The drawing under review shows one solid part. Ordinate dimensions are in mm from its lowest x, y, z. A direction names the side the tool comes from. Give positions to 0.01 mm unless a question says otherwise; leave off trailing zeros. Order: outer loops, then holes, each group sorted by start corner. A loop starts at its lowest first (then second) coordinate and runs counter-clockwise, first axis right, second up. Notation, with made-up numbers: (50.5, -21) - (94.5, -21) arc R25 cw to (94.5, 17) - close; hole circle Ø8 at (33.25, 8). An arc over 180 degrees is marked (long way). Write item = value, one per line. Start each with the question number.
1. Wall thickness on probe 1 along X at (y, z) = (3.75, 15.65); probe 2 along Z at (x, y) = (25, 6); probe 3 along Z at (x, y) = (11.5, 4.75): over which ranges is each line inside the solid? List them lowest first.
2. We need section C-C, the plane y = 4.25. State how many separate pieces and enclosed holes the cut face has.
3. Mouldability with a two-part tool opening along Z and no side actions: class the marked faces 5, 6 and 7 as pulls with the +Z half, pulls with the -Z half, needs draft (parallel to the pull), parting line crosses it, or undercut.
4. Machinability: for the marked faces 1, 2, 3 and 4, which of the approach directions +Z, -Z, +X, -X, +Y, -Y give a long, thin tool a straight path to every point of the face, cutting with its end or side? Answer none if there is none.
5. We need section D-D, the plane z = 8.5. Give the boundary of the cut face in (x, y).
6. We need section B-B, the plane z = 5.35. Give the boundary of the cut face in (x, y), and give its area (3 significant figures).
7. We need section A-A, the plane x = 25.1. Give the boundary of the cut face in (y, z).
8. For P1, Ø1.5, axis at x = 31, y = 1, coming from the -Z side; P2, Ø6, axis at y = 3.5, z = 4.5, coming from the +X side; P3, Ø1.6, axis at y = 5.5, z = 1.5, coming from the -X side, all flat-tipped, find the tip position at first contact; note any pin that passes through.
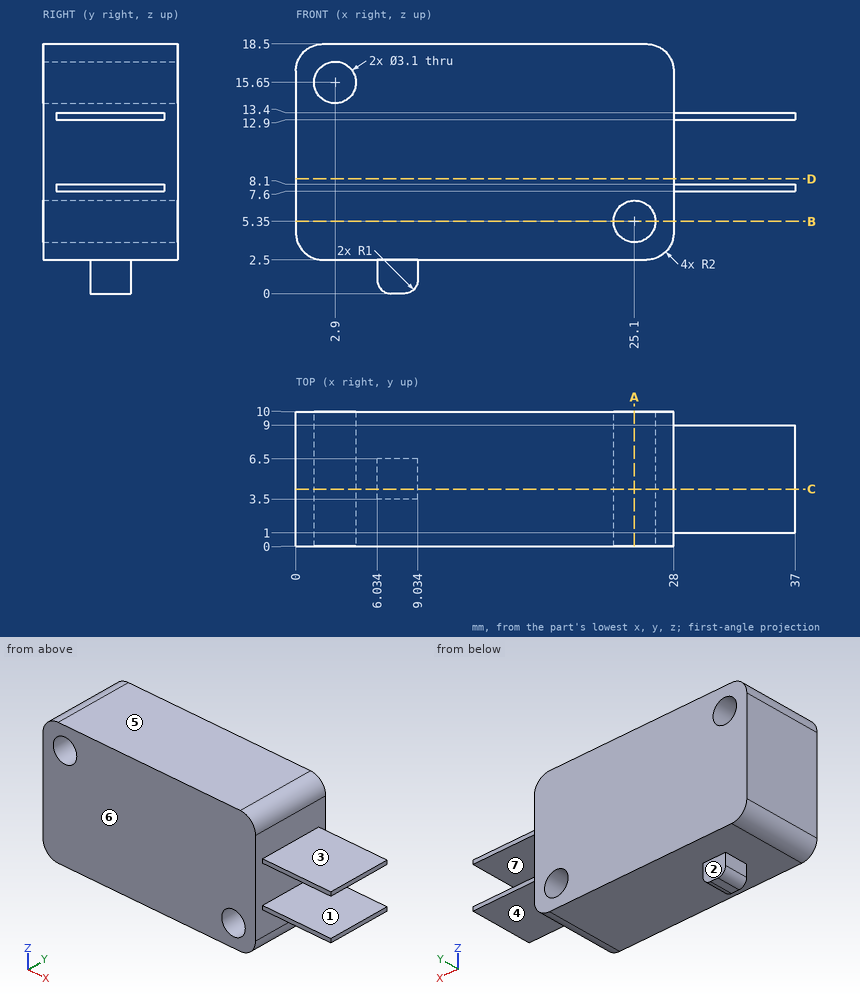
Model answer:
q1.probe_1 = 0 to 1.35, 4.45 to 28
q1.probe_2 = 2.5 to 3.8, 6.9 to 18.5
q1.probe_3 = 2.5 to 18.5
q2.separate_pieces = 1
q2.enclosed_holes = 2
q3.face_5 = pulls with the +Z half
q3.face_6 = needs draft
q3.face_7 = undercut
q4.face_1 = +X, +Y, -Y
q4.face_2 = -Z, +X, -X, +Y
q4.face_3 = +Z, +X, +Y, -Y
q4.face_4 = -Z, +X, +Y, -Y
q5.outline = (0, 0) - (28, 0) - (28, 10) - (0, 10) - close
q6.outline = (0, 0) - (23.55, 0) - (23.55, 10) - (0, 10) - close; (26.65, 0) - (28, 0) - (28, 10) - (26.65, 10) - close
q6.area = 249 mm2
q7.outline = (0, 2.5) - (10, 2.5) - (10, 3.8) - (0, 3.8) - close; (0, 6.9) - (10, 6.9) - (10, 18.5) - (0, 18.5) - close
q8.P1 = 7.6
q8.P2 = 28
q8.P3 = 6.03
